```python
from build123d import *

# Parameters (mm, degrees)
SKETCH_1_W          = 50
SKETCH_1_H          = 40
EXTRUDE_1_DEPTH     = 10
SKETCH_2_R          = 1
CUT_EXTRUDE_1_DEPTH = 34.541019662
SKETCH_10_R         = 1.85
CUT_EXTRUDE_6_DEPTH = 2
SKETCH_11_W         = 26
SKETCH_11_H         = 6
CUT_EXTRUDE_7_DEPTH = 6.3
SKETCH_13_R         = 1.45
CUT_EXTRUDE_8_DEPTH = 10


with BuildPart() as part:
    # 草图1 → 凸台-拉伸1 (new body)
    with BuildSketch(Plane.XY):
        Rectangle(SKETCH_1_W, SKETCH_1_H)
    extrude(amount=EXTRUDE_1_DEPTH)

    # 草图2 → 切除-拉伸1 (cut, through all)
    with BuildSketch(Plane.XY.offset(10)):
        with Locations((-9.648315915, 10)):
            Circle(SKETCH_2_R)
        with Locations((9.751684085, 10)):
            Circle(SKETCH_2_R)
    extrude(amount=-CUT_EXTRUDE_1_DEPTH, mode=Mode.SUBTRACT)

    # 草图10 → 切除-拉伸6 (cut)
    with BuildSketch(Plane.XY.offset(10)):
        with Locations((-9.648315915, 10)):
            Circle(SKETCH_10_R)
        with Locations((9.751684085, 10)):
            Circle(SKETCH_10_R)
    extrude(amount=-CUT_EXTRUDE_6_DEPTH, mode=Mode.SUBTRACT)

    # 草图11 → 切除-拉伸7 (cut)
    with BuildSketch(Plane(origin=(0, 0, 0), x_dir=(-1, 0, 0), z_dir=(0, 0, -1))):
        with Locations((0, 10)):
            Rectangle(SKETCH_11_W, SKETCH_11_H)
    extrude(amount=-CUT_EXTRUDE_7_DEPTH, mode=Mode.SUBTRACT)

    # 草图13 → 切除-拉伸8 (cut)
    with BuildSketch(Plane.XY.offset(10)):
        with Locations((-16.023529812, 16)):
            Circle(SKETCH_13_R)
        with Locations((-16.023529812, -16)):
            Circle(SKETCH_13_R)
        with Locations((15.976470188, 16)):
            Circle(SKETCH_13_R)
        with Locations((15.976470188, -16)):
            Circle(SKETCH_13_R)
    extrude(amount=-CUT_EXTRUDE_8_DEPTH, mode=Mode.SUBTRACT)


solid = part.part
```
The model under review builds one solid part; all positions refer to its coordinate system, in mm. A direction names the side the tool comes from. Give positions to 0.01 mm unless a question says otherwise; leave off trailing zeros. Write each loop counter-clockwise with the first axis right and the second up, starting at its lowest first coordinate (ties: lowest second). Pieces come first, ordered by that corner, then holes.
(1) Consider section B-B, the plane z = 1. Give the boundary of the cut face in (x, y), and give its area (3 significant figures).
(2) Consider section D-D, the plane y = 10. Give the boundary of the cut face in (x, z), and give its area (3 significant figures).
(3) Consider section C-C, the plane x = -1. Give the boundary of the cut face in (y, z).
(4) To check wall thickness, follow L1, parallel to Y at x = 2.5, z = 2.75. State the ranges of the line that lie inside material, in increasing order.
(5) Tool access review of faces 4 (the flat face through (13, 10, 3)), 5 (the flat face through (0, 20, 5)), 6 (the flat face through (11, 9, 8)): name each direction out of +Z, -Z, +X, -X, +Y, -Y from which nothing blocks a thin tool from reaching the whole face with its end or side.
(6) Consider section A-A, the plane y = -16. Give the boundary of the cut face in (x, z).
(7) For P1, Ø3.5, axis at x = 9.75, y = 10, coming from the +Z side; P2, Ø1.5, axis at x = -0.5, y = 9.5, coming from the -Z side; P3, Ø1.2, axis at x = 9.75, y = 10, coming from the -Z side, all flat-tipped, find the tip position at first contact; note any pin that passes through.
(8) The part is to be moulded in two halves that separate along X. For faces 1 (the flat face through (25, 0, 5)), 2 (the cylindrical face through (8.284, 8.874, 9.014)), 3 (the flat face through (0, 0, 0)), say which applies: released by +X, released by -X, zero draft, split by the parting line, or undercut.
Returned:
1. outline: (-25, -20) - (25, -20) - (25, 20) - (-25, 20) - close; hole circle Ø2.9 at (-16.02, -16); hole circle Ø2.9 at (-16.02, 16); hole (-13, 7) - (13, 7) - (13, 13) - (-13, 13) - close; hole circle Ø2.9 at (15.98, -16); hole circle Ø2.9 at (15.98, 16)
1. area: 1,820 mm2
2. outline: (-25, 0) - (-13, 0) - (-13, 6.3) - (-10.65, 6.3) - (-10.65, 8) - (-11.5, 8) - (-11.5, 10) - (-25, 10) - close; (-8.65, 6.3) - (8.75, 6.3) - (8.75, 8) - (7.9, 8) - (7.9, 10) - (-7.8, 10) - (-7.8, 8) - (-8.65, 8) - close; (10.75, 6.3) - (13, 6.3) - (13, 0) - (25, 0) - (25, 10) - (11.6, 10) - (11.6, 8) - (10.75, 8) - close
2. area: 315 mm2
3. outline: (-20, 0) - (7, 0) - (7, 6.3) - (13, 6.3) - (13, 0) - (20, 0) - (20, 10) - (-20, 10) - close
4. L1: y = -20 to 7, 13 to 20
5. face 4: -Z
5. face 5: +Z, -Z, +X, -X, +Y
5. face 6: +Z
6. outline: (-25, 0) - (-17.47, 0) - (-17.47, 10) - (-25, 10) - close; (-14.57, 0) - (14.53, 0) - (14.53, 10) - (-14.57, 10) - close; (17.43, 0) - (25, 0) - (25, 10) - (17.43, 10) - close
7. P1: stops at z = 8
7. P2: stops at z = 6.3
7. P3: passes through
8. face 1: released by +X
8. face 2: undercut
8. face 3: zero draft
